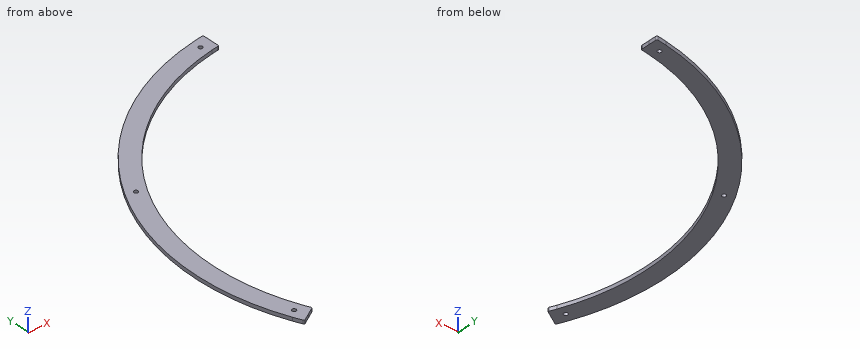
from build123d import *

# Parameters (mm, degrees)
PAD021_DEPTH                        = 3
SKETCH083_R                         = 1.7
POCKET041_DEPTH                     = 0.001
POCKET041_DEPTH_BACK                = 3.001
SKETCH084_R                         = 1.7
POCKET042_DEPTH                     = 0.001
POCKET042_DEPTH_BACK                = 3.001
BODY001003005003013_PLACEMENT_ANGLE = 60


with BuildPart() as part:
    # Sketch082 → Pad021 (new body)
    with BuildSketch(Plane.XY):
        with BuildLine():
            ThreePointArc((156.627412, 120.879551), (87.258751, 177.56667), (0, 197.848457))
            Line((0, 197.848457), (0, 182.848457))
            ThreePointArc((144.752611, 111.714995), (80.643177, 164.104346), (0, 182.848457))
            ThreePointArc((148.102078, 107.234942), (146.444477, 109.487778), (144.752611, 111.714995))
            ThreePointArc((148.102078, 107.234942), (148.703343, 106.843433), (149.41205, 106.955386))
            Line((155.154429, 110.27075), (149.41205, 106.955386))
            Line((155.154429, 110.27075), (160.726477, 113.487773))
            ThreePointArc((160.726477, 113.487773), (161.203737, 114.141753), (161.040435, 114.934722))
            ThreePointArc((161.040435, 114.934722), (158.861734, 117.927781), (156.627412, 120.879551))
        make_face()
    pad021 = extrude(amount=PAD021_DEPTH)

    # Mirrored029: Pad021 across Sketch082 V_Axis
    add(pad021.mirror(Plane(origin=(0, 0, 0), x_dir=(0, 0, 1), z_dir=(1, 0, 0))))

    # Sketch083 → Pocket041 (cut, two sides)
    with BuildSketch(Plane.XY) as pocket041_sk:
        with Locations((149.149219, 118.266841)):
            Circle(SKETCH083_R)
        with Locations((-149.149219, 118.266841)):
            Circle(SKETCH083_R)
    extrude(amount=-POCKET041_DEPTH, mode=Mode.SUBTRACT)
    extrude(pocket041_sk.sketch, amount=POCKET041_DEPTH_BACK, mode=Mode.SUBTRACT)

    # Sketch084 → Pocket042 (cut, two sides)
    with BuildSketch(Plane.XY) as pocket042_sk:
        with Locations((0, 190.348457)):
            Circle(SKETCH084_R)
    extrude(amount=-POCKET042_DEPTH, mode=Mode.SUBTRACT)
    extrude(pocket042_sk.sketch, amount=POCKET042_DEPTH_BACK, mode=Mode.SUBTRACT)


with BuildPart() as part_1:
    # Body001003005003013 placement: moved
    add(part.part.rotate(Axis((0, 0, 0), (0, 0, 1)), BODY001003005003013_PLACEMENT_ANGLE))


solid = part_1.part
For this review, take the finished solid that the model builds, in its own axes (mm). Give positions to 0.01 mm unless a question says otherwise; leave off trailing zeros. Loops run counter-clockwise (first coordinate to the right, second up) from the corner with the lowest first, then second, coordinate; pieces in that order, holes last. Notation, with made-up numbers: (-27, 65.25) - (27, 65.25) arc R24 ccw to (27, 79.25) - close; hole circle Ø2 at (43.25, 33). An arc over 180 degrees is marked (long way). Write each question's results on one line, items separated by ' | '.
(1) Take a section at A-A (z = 1.85). Give the boundary of the cut face in (x, y), then the cut area to 3 significant figures.
Conclusion:
outline: (-183, -75.2) arc R197.85 ccw to (-180.06, -82) arc R1 ccw to (-178.65, -82.45) - (-167.33, -75.92) arc R1 ccw to (-166.92, -74.64) arc R182.85 cw to (-169.12, -69.5) arc R182.85 cw to (-158.35, 91.42) arc R182.85 cw to (-24.37, 181.22) arc R182.85 cw to (-18.82, 181.88) arc R1 ccw to (-17.92, 182.87) - (-17.92, 195.94) arc R1 ccw to (-19.02, 196.93) arc R197.85 ccw to (-26.37, 196.08) arc R197.85 ccw to start; hole circle Ø3.4 at (-177, -70.03); hole circle Ø3.4 at (-164.85, 95.17); hole circle Ø3.4 at (-27.85, 188.3) | area: 5,410 mm^2
(2) Take a section at C-C (y = -50.5). Give the boundary of the cut face in (x, z).
Conclusion:
outline: (-191.29, 0) - (-175.74, 0) - (-175.74, 3) - (-191.29, 3) - close
(3) Take a section at B-B (x = -52). Give the boundary of the cut face in (y, z), then the cut area to 3 significant figures.
Conclusion:
outline: (175.3, 0) - (190.89, 0) - (190.89, 3) - (175.3, 3) - close | area: 46.8 mm^2
(4) For line 1 along X through (y, z) = (-1, 0.4); line 2 along X through (y, z) = (96.5, 0.4); line 3 along X through (y, z) = (-25.5, 2.8), list the stretches that pass through material, from the lowest coordinate up.
Conclusion:
line 1: -197.85 to -182.85 | line 2: -172.72 to -165.91, -163.78 to -155.31 | line 3: -196.2 to -181.06
(5) For pin 1 Ø2 at (x, y) = (-27.85, 188.3) entering from +Z; pin 2 Ø1.5 at (x, z) = (-48, 2) entering from +Y, all flat-tipped, find the tip position at first contact; note any pin that passes through.
Conclusion:
pin 1: through | pin 2: y = 192.12
